For this review, take the finished solid that the model builds, in its own axes (mm). Face numbers are marked on the shaded views. A direction names the side the tool comes from. Give positions to 0.01 mm unless a question says otherwise; leave off trailing zeros. Order: outer loops, then holes, each group sorted by start corner. A loop starts at its lowest first (then second) coordinate and runs counter-clockwise, first axis right, second up. Notation, with made-up numbers: (18, 54) - (40, 54) arc R31 cw to (40, 89) - close; hole circle Ø3 at (59, 30). An arc over 180 degrees is marked (long way). One line per item, written item: value.
Autodesk Inventor part; units mm, degrees
ref_plane "YZ Plane" through (0, 0, 0) normal (1, 0, 0) x (0, 1, 0)
ref_plane "XZ Plane" through (0, 0, 0) normal (0, 1, 0) x (-1, 0, 0)
ref_plane "XY Plane" through (0, 0, 0) normal (0, 0, 1) x (1, 0, 0)
sketch "Sketch1" plane through (0, 0, 0) normal (0, 1, 0) x (-1, 0, 0)
  circle A0 centre (0, 0) radius 45
  dimension "d0" = 90
extrude "Extrusion1" add sketch "Sketch1" along normal blind 10
sketch "Sketch2" plane through (0, 0, 0) normal (0, -1, 0) x (1, 0, 0)
  circle A0 centre (0, 0) radius 26
  dimension "d3" = 52
extrude "Extrusion2" add sketch "Sketch2" along normal blind 28
sketch "Sketch3" plane through (0, -28, 0) normal (0, -1, 0) x (1, 0, 0)
  circle A0 centre (0, 0) radius 21
  dimension "d6" = 42
extrude "Extrusion3" cut sketch "Sketch3" against normal blind 28
sketch "Sketch4" plane through (0, -28, 0) normal (0, -1, 0) x (1, 0, 0)
  circle A0 centre (0, 0) radius 22.1
  circle A1 centre (0, 0) radius 24.8
  dimension "d9" = 44.2
  dimension "d10" = 49.6
extrude "Extrusion4" cut sketch "Sketch4" against normal blind 2.2
sketch "Sketch5" plane through (0, 0, 0) normal (0, -1, 0) x (1, 0, 0)
  point P0 (0, 0)
  point P1 (0, 0)
hole "Hole1" at (0, 0, 0) direction (0, 1, 0) diameter 29.8349 end through all
sketch "Sketch6" plane through (0, 0, 0) normal (0, -1, 0) x (1, 0, 0)
  point P0 (0, 0)
  point P1 (0, 37.5)
  point P2 (-26.5165, 26.5165)
  point P3 (-37.5, 0)
  point P4 (-26.5165, -26.5165)
  point P5 (0, -37.5)
  point P6 (26.5165, -26.5165)
  point P7 (37.5, 0)
  point P8 (26.5165, 26.5165)
  dimension "d20" = 37.5
  dimension "d30" = 360
hole "Hole2" at (0, 0, 37.5) at (-26.5165, 0, 26.5165) at (-37.5, 0, 0) at (-26.5165, 0, -26.5165) at (0, 0, -37.5) at (26.5165, 0, -26.5165) at (37.5, 0, 0) at (26.5165, 0, 26.5165) direction (0, 1, 0) diameter 5.5 end through all countersink diameter 10.4 countersink angle 90
properties part number "Passthrough Base"
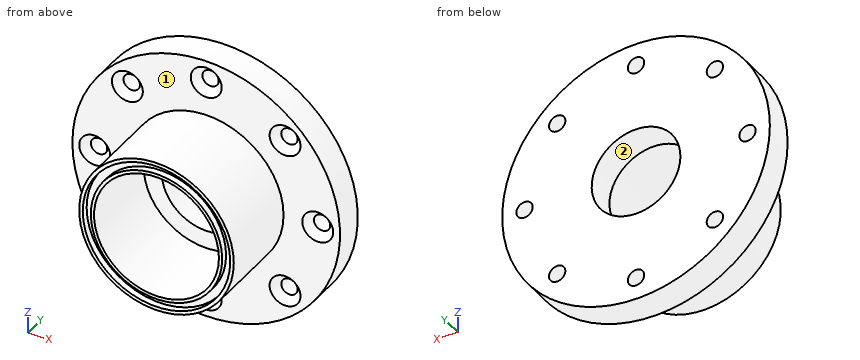
(1) Wall thickness on line 1 (Z direction, x = 0, y = 5); line 2 (X direction, y = -19, z = -1); line 3 (Z direction, x = 0, y = -19): over which ranges is each line inside the solid? List them lowest first. Write a range as from..to.
Answers below:
line 1: z = -45..-40.25, -34.75..-14.92, 14.92..34.75, 40.25..45
line 2: x = -25.98..-20.98, 20.98..25.98
line 3: z = -26..-21, 21..26
(2) Take a section at B-B (z = 37.5). Write out the cut boundary in (x, y).
Answers below:
outline: (-24.87, 0) - (-5.2, 0) - (-2.75, 2.45) - (-2.75, 10) - (-24.87, 10) - close; (2.75, 2.45) - (5.2, 0) - (24.87, 0) - (24.87, 10) - (2.75, 10) - close
(3) For P1, Ø5, axis at x = 26.52, z = 26.52, coming from the -Y side; P2, Ø2, axis at y = -12, z = -15, coming from the +X side; P3, Ø25, axis at x = 8.5, z = 6, coming from the -Y side; P4, Ø12, axis at y = -17, z = 10, coming from the +X side, all flat-tipped, find the tip position at first contact; note any pin that passes through.
Answers below:
P1: passes through
P2: stops at x = 21.91
P3: stops at y = -28
P4: stops at x = 25.69
(4) Machinability: for the marked faces 1 and 2, which of the approach directions +Z, -Z, +X, -X, +Y, -Y give a long, thin tool a straight path to every point of the face, cutting with its end or side? Answer none if there is none.
Answers below:
face 1: -Y
face 2: +Y, -Y
(5) Take a section at D-D (y = -17). Write out the cut boundary in (x, z), then the cut area to 3 significant figures.
Answers below:
outline: circle Ø52 at (0, 0); hole circle Ø42 at (0, 0)
area: 738 mm^2
(6) Take a section at A-A (x = 37.5). Write out the cut boundary in (y, z).
Answers below:
outline: (0, -24.87) - (10, -24.87) - (10, -2.75) - (2.45, -2.75) - (0, -5.2) - close; (0, 5.2) - (2.45, 2.75) - (10, 2.75) - (10, 24.87) - (0, 24.87) - close
(7) Take a section at C-C (y = 6). Give the number of separate pieces and of enclosed holes in the cut face, then the cut area to 3 significant figures.
Answers below:
separate pieces: 1
enclosed holes: 9
area: 5,470 mm^2
